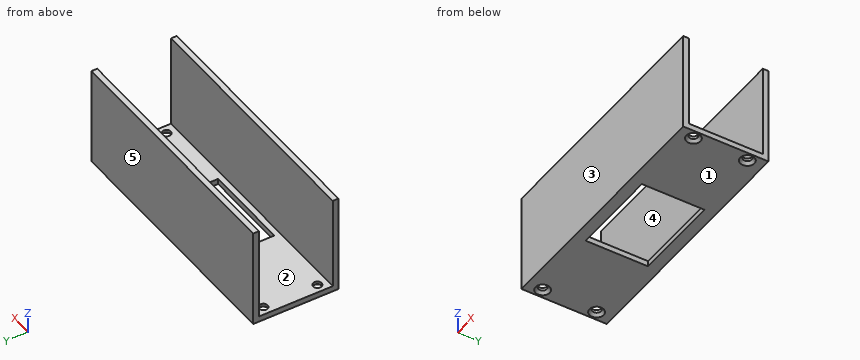
```python
from build123d import *

# Parameters (mm, degrees)
SKETCH_W     = 89
SKETCH_H     = 30
PAD_DEPTH    = 2
SKETCH001_W  = 89
SKETCH001_H  = 2
PAD001_DEPTH = 33
SKETCH002_R  = 1.5
SKETCH002_W  = 31
SKETCH002_H  = 22
POCKET_DEPTH = 2
CHAMFER_SIZE = 1


with BuildPart() as part:
    # Sketch → Pad (new body)
    with BuildSketch(Plane.XY):
        Rectangle(SKETCH_W, SKETCH_H)
    extrude(amount=PAD_DEPTH)

    # Sketch001 (on Face6 of Pad) → Pad001 (join)
    with BuildSketch(Plane.XY.offset(2)):
        with Locations((0, 14)):
            Rectangle(SKETCH001_W, SKETCH001_H)
        with Locations((0, -14)):
            Rectangle(SKETCH001_W, SKETCH001_H)
    extrude(amount=PAD001_DEPTH)

    # Sketch002 (on Face8 of Pad001) → Pocket (cut)
    with BuildSketch(Plane.XY.offset(2)):
        with Locations((41.5, 9.5)):
            Circle(SKETCH002_R)
        with Locations((41.5, -9.5)):
            Circle(SKETCH002_R)
        with Locations((-41.5, -9.5)):
            Circle(SKETCH002_R)
        with Locations((-41.5, 9.5)):
            Circle(SKETCH002_R)
        Rectangle(SKETCH002_W, SKETCH002_H)
    extrude(amount=-POCKET_DEPTH, mode=Mode.SUBTRACT)

    # Chamfer
    chamfer_edges = [part.edges().sort_by_distance(p)[0] for p in [
        (-43, 9.5, 0),
        (-43, -9.5, 0),
        (40, -9.5, 0),
        (40, 9.5, 0),
    ]]
    chamfer(chamfer_edges, length=CHAMFER_SIZE)


solid = part.part
```
Work out the finished part from the listing and answer in its coordinate system (mm). Face numbers are marked on the shaded views. A direction names the side the tool comes from. Round coordinates to 2 decimals unless told otherwise and drop trailing zeros. Write each loop counter-clockwise with the first axis right and the second up, starting at its lowest first coordinate (ties: lowest second). Pieces come first, ordered by that corner, then holes. Notation, with made-up numbers: (-14.5, 23.5) -> (24.5, 23.5) arc R16 ccw to (24.5, 52.5) -> close; hole circle Ø6 at (20.25, -23). An arc over 180 degrees is marked (long way). Write each question's results on one line, items separated by ' | '.
Q1. Determine the mould class of the marked faces 3, 4 and 5 for opening direction Y: released by +Y, released by -Y, zero draft, split by the parting line, or undercut.
Data:
face 3: released by -Y | face 4: undercut | face 5: released by +Y
Q2. Flat-ended cylindrical pins translate along their axes: P1, Ø1.8, axis at x = -41.5, y = 9.5, coming from the -Z side; P2, Ø13, axis at x = 18, y = -3.5, coming from the +Z side. Find the tip coordinate at first contact, or state that the pin passes through.
Data:
P1: through | P2: z = 2
Q3. Straight lines are drawn through the part: line 1 along Y through (x, z) = (41.5, 1.55); line 2 along Y through (x, z) = (41, 1); line 3 along Y through (x, z) = (-32, 14). For each, find the intervals that lie inside material, in ascending order. Write a range as [from, to].
Data:
line 1: [-15, -11], [-8, 8], [11, 15] | line 2: [-15, -10.91], [-8.09, 8.09], [10.91, 15] | line 3: [-15, -13], [13, 15]
Q4. Section B-B, the plane x = 41.5 is taken. Write down the section's boundary in (y, z).
Data:
outline: (-15, 0) -> (-12, 0) -> (-11, 1) -> (-11, 2) -> (-13, 2) -> (-13, 35) -> (-15, 35) -> close; (-8, 1) -> (-7, 0) -> (7, 0) -> (8, 1) -> (8, 2) -> (-8, 2) -> close; (11, 1) -> (12, 0) -> (15, 0) -> (15, 35) -> (13, 35) -> (13, 2) -> (11, 2) -> close
Q5. Section D-D, the plane x = -14 is taken. Write down the section's boundary in (y, z), then the cut area to 3 significant figures.
Data:
outline: (-15, 0) -> (-11, 0) -> (-11, 2) -> (-13, 2) -> (-13, 35) -> (-15, 35) -> close; (11, 0) -> (15, 0) -> (15, 35) -> (13, 35) -> (13, 2) -> (11, 2) -> close | area: 148 mm^2
Q6. Section A-A, the plane y = 9.5 is taken. Write down the section's boundary in (x, z).
Data:
outline: (-44.5, 0) -> (-44, 0) -> (-43, 1) -> (-43, 2) -> (-44.5, 2) -> close; (-40, 1) -> (-39, 0) -> (-15.5, 0) -> (-15.5, 2) -> (-40, 2) -> close; (15.5, 0) -> (39, 0) -> (40, 1) -> (40, 2) -> (15.5, 2) -> close; (43, 1) -> (44, 0) -> (44.5, 0) -> (44.5, 2) -> (43, 2) -> close
Q7. Section C-C, the plane z = 17 is taken. Write down the section's boundary in (x, y), then the cut area to 3 significant figures.
Data:
outline: (-44.5, -15) -> (44.5, -15) -> (44.5, -13) -> (-44.5, -13) -> close; (-44.5, 13) -> (44.5, 13) -> (44.5, 15) -> (-44.5, 15) -> close | area: 356 mm^2
Q8. Which of the six approach directions +Z, -Z, +X, -X, +Y, -Y give full straight-line access (tool end or side, diameter ignored) to the marked faces 1 and 2?
Data:
face 1: -Z, +X, -X, +Y, -Y | face 2: +Z, +X, -X
